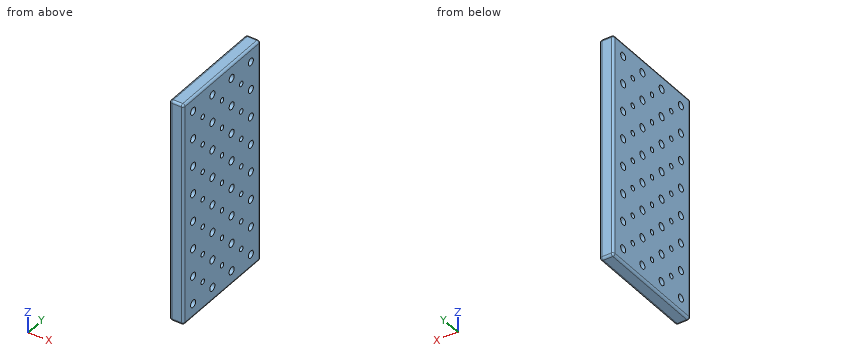
Autodesk Inventor part; units mm, degrees
ref_plane "YZ Plane" through (0, 0, 0) normal (1, 0, 0) x (0, 1, 0)
ref_plane "XZ Plane" through (0, 0, 0) normal (0, 1, 0) x (-1, 0, 0)
ref_plane "XY Plane" through (0, 0, 0) normal (0, 0, 1) x (1, 0, 0)
sketch "fourth" plane through (0, 0, 0) normal (1, 0, 0) x (0, 1, 0)
  line L0 (50, 100) -> (50, 0)
  line L1 (50, 100) -> (0, 100)
  line L2 (0, 75) -> (0, 100)
  line L3 (0, 75) -> (0, 50)
  line L4 (0, 50) -> (0, 25)
  line L5 (0, 25) -> (0, 0)
  line L6 (25, 75) -> (0, 75)
  line L7 (25, 75) -> (25, 50)
  line L8 (25, 50) -> (25, 25)
  line L9 (25, 25) -> (25, 0)
  line L10 (37.5, 87.5) -> (37.5, 62.5)
  line L11 (37.5, 62.5) -> (37.5, 37.5)
  line L12 (37.5, 37.5) -> (37.5, 12.5)
  line L13 (12.5, 87.5) -> (37.5, 87.5)
  line L14 (12.5, 87.5) -> (12.5, 62.5)
  line L15 (12.5, 62.5) -> (12.5, 37.5)
  line L16 (12.5, 37.5) -> (12.5, 12.5)
  line L17 (50, -100) -> (50, 0)
  line L18 (50, -100) -> (0, -100)
  line L19 (0, -75) -> (0, -100)
  line L20 (0, -75) -> (0, -50)
  line L21 (0, -50) -> (0, -25)
  line L22 (0, -25) -> (0, 0)
  line L23 (25, -75) -> (0, -75)
  line L24 (25, -75) -> (25, -50)
  line L25 (25, -50) -> (25, -25)
  line L26 (25, -25) -> (25, 0)
  line L27 (37.5, -87.5) -> (37.5, -62.5)
  line L28 (37.5, -62.5) -> (37.5, -37.5)
  line L29 (37.5, -37.5) -> (37.5, -12.5)
  line L30 (12.5, -87.5) -> (37.5, -87.5)
  line L31 (12.5, -87.5) -> (12.5, -62.5)
  line L32 (12.5, -62.5) -> (12.5, -37.5)
  line L33 (12.5, -37.5) -> (12.5, -12.5)
  line L34 (-50, 100) -> (-50, 0)
  line L35 (-50, 100) -> (0, 100)
  line L36 (-25, 75) -> (0, 75)
  line L37 (-25, 75) -> (-25, 50)
  line L38 (-25, 50) -> (-25, 25)
  line L39 (-25, 25) -> (-25, 0)
  line L40 (-37.5, 87.5) -> (-37.5, 62.5)
  line L41 (-37.5, 62.5) -> (-37.5, 37.5)
  line L42 (-37.5, 37.5) -> (-37.5, 12.5)
  line L43 (-12.5, 87.5) -> (-37.5, 87.5)
  line L44 (-12.5, 87.5) -> (-12.5, 62.5)
  line L45 (-12.5, 62.5) -> (-12.5, 37.5)
  line L46 (-12.5, 37.5) -> (-12.5, 12.5)
  line L47 (-25, -75) -> (-25, -50)
  line L48 (-25, -75) -> (0, -75)
  line L49 (-37.5, -87.5) -> (-37.5, -62.5)
  line L50 (-12.5, -87.5) -> (-12.5, -62.5)
  line L51 (-50, -100) -> (0, -100)
  line L52 (-12.5, -87.5) -> (-37.5, -87.5)
  line L53 (-37.5, -62.5) -> (-37.5, -37.5)
  line L54 (-12.5, -62.5) -> (-12.5, -37.5)
  line L55 (-50, -100) -> (-50, 0)
  line L56 (-25, -50) -> (-25, -25)
  line L57 (-37.5, -37.5) -> (-37.5, -12.5)
  line L58 (-12.5, -37.5) -> (-12.5, -12.5)
  line L59 (-25, -25) -> (-25, 0)
  dimension "d16" = 50
  dimension "d22" = 100
  dimension "d23" = 100
  dimension "d24" = 25
  dimension "d25" = 12.5
  dimension "d26" = 12.5
extrude "Extrusion1" add sketch "fourth" along normal blind 12.5
hole "Hole1" at (0, 25, 75) at (0, 25, 50) at (0, 25, 25) at (0, 25, 0) at (0, 25, -25) at (0, 25, -50) at (0, 25, -75) at (0, 0, 75) at (0, 0, 50) at (0, -25, 75) at (0, -25, 50) at (0, -25, 25) at (0, -25, 0) at (0, -25, -25) at (0, -25, -50) at (0, -25, -75) at (0, 0, -75) at (0, 0, -50) at (0, 0, -25) at (0, 0, 0) at (0, 0, 25) direction (1, 0, 0) diameter 4.5 end through all
hole "Hole2" at (0, 37.5, 87.5) at (0, 37.5, 62.5) at (0, 37.5, 37.5) at (0, 37.5, 12.5) at (0, 12.5, 87.5) at (0, 12.5, 62.5) at (0, 12.5, 37.5) at (0, 12.5, 12.5) at (0, 37.5, -87.5) at (0, 37.5, -62.5) at (0, 12.5, -87.5) at (0, 12.5, -62.5) at (0, 37.5, -37.5) at (0, 12.5, -37.5) at (0, 37.5, -12.5) at (0, 12.5, -12.5) at (0, -37.5, 87.5) at (0, -37.5, 62.5) at (0, -37.5, 37.5) at (0, -37.5, 12.5) at (0, -12.5, 37.5) at (0, -12.5, 12.5) at (0, -12.5, 62.5) at (0, -12.5, 87.5) at (0, -37.5, -37.5) at (0, -37.5, -12.5) at (0, -12.5, -37.5) at (0, -12.5, -12.5) at (0, -37.5, -62.5) at (0, -12.5, -62.5) at (0, -12.5, -87.5) at (0, -37.5, -87.5) direction (1, 0, 0) diameter 6.5 end through all
fillet "Fillet1" radius 2 12 edges at (12.5, 0, 100) (12.5, 50, 0) (12.5, 0, -100) (12.5, -50, 0) (0, 50, 0) (0, 0, 100) (0, -50, 0) (0, 0, -100) (6.25, 50, -100) (6.25, 50, 100) (6.25, -50, 100) (6.25, -50, -100)
properties part number "Base_Plate" material "Titanium"
Here's how the part is built. I have some questions about the finished solid (model axes, mm). Round coordinates to 2 decimals unless told otherwise and drop trailing zeros. Order: outer loops, then holes, each group sorted by start corner. A loop starts at its lowest first (then second) coordinate and runs counter-clockwise, first axis right, second up. Notation, with made-up numbers: (-40, 15.25) -> (17, 15.25) arc R16 cw to (17, 40.25) -> close; hole circle Ø7 at (-11.5, -31.5). An arc over 180 degrees is marked (long way). Use a Markdown table: item, result. Add a question column.
(1) I need wall thicknesses on line 1 along Y through (x, z) = (7, -75); line 2 along Y through (x, z) = (9.75, 37.5); line 3 along Y through (x, z) = (11.5, -48.5). Which ranges of each line are inside material? Lowest first, please.
(2) Suppose I cut it at C-C, the plane y = -37.5. Count the separate pieces of the cut face and the enclosed holes in it, and give its area (3 significant figures).
(3) Suppose I cut it at A-A, the plane z = 62.5. Please give me the cut outline in (x, y), and give its area (3 significant figures).
(4) Suppose I cut it at B-B, the plane z = -75. Please give me the cut outline in (x, y), and give its area (3 significant figures).
Verdict:
| question | item | result |
|---|---|---|
| 1 | line 1 | -50 to -27.25, -22.75 to -2.25, 2.25 to 22.75, 27.25 to 50 |
| 1 | line 2 | -50 to -40.75, -34.25 to -15.75, -9.25 to 9.25, 15.75 to 34.25, 40.75 to 50 |
| 1 | line 3 | -49.73 to -26.68, -23.32 to -1.68, 1.68 to 23.32, 26.68 to 49.73 |
| 2 | separate pieces | 9 |
| 2 | enclosed holes | 0 |
| 2 | area | 1,850 mm2 |
| 3 | outline | (0, -48) arc R2 ccw to (2, -50) -> (10.5, -50) arc R2 ccw to (12.5, -48) -> (12.5, -40.75) -> (0, -40.75) -> close; (0, -34.25) -> (12.5, -34.25) -> (12.5, -15.75) -> (0, -15.75) -> close; (0, -9.25) -> (12.5, -9.25) -> (12.5, 9.25) -> (0, 9.25) -> close; (0, 15.75) -> (12.5, 15.75) -> (12.5, 34.25) -> (0, 34.25) -> close; (0, 40.75) -> (12.5, 40.75) -> (12.5, 48) arc R2 ccw to (10.5, 50) -> (2, 50) arc R2 ccw to (0, 48) -> close |
| 3 | area | 922 mm2 |
| 4 | outline | (0, -48) arc R2 ccw to (2, -50) -> (10.5, -50) arc R2 ccw to (12.5, -48) -> (12.5, -27.25) -> (0, -27.25) -> close; (0, -22.75) -> (12.5, -22.75) -> (12.5, -2.25) -> (0, -2.25) -> close; (0, 2.25) -> (12.5, 2.25) -> (12.5, 22.75) -> (0, 22.75) -> close; (0, 27.25) -> (12.5, 27.25) -> (12.5, 48) arc R2 ccw to (10.5, 50) -> (2, 50) arc R2 ccw to (0, 48) -> close |
| 4 | area | 1,080 mm2 |
